Can you work these out from the model? Positions are in its coordinate system, mm. Give positions to 0.01 mm unless a question says otherwise; leave off trailing zeros. Order: outer loops, then holes, each group sorted by start corner. A loop starts at its lowest first (then second) coordinate and runs counter-clockwise, first axis right, second up. Notation, with made-up numbers: (10.5, -14.5) - (40.5, -14.5) arc R11 cw to (40.5, 0.5) - close; hole circle Ø2 at (23.25, 72). An arc over 180 degrees is marked (long way). One line per question, with ' | ' between items.
```python
from build123d import *

# Parameters (mm, degrees)
CYLINDER_R          = 1.5
CYLINDER_DEPTH      = 10
CYLINDER_ROLL_ANGLE = 90
CUT_PLACEMENT_ANGLE = 180


with BuildPart() as cylinder:
    # Cylinder → Cylinder (new body)
    with BuildSketch(Plane.XY):
        Circle(CYLINDER_R)
    extrude(amount=CYLINDER_DEPTH)


with BuildPart() as cylinder_1:
    # Cylinder roll: moved
    add(cylinder.part.rotate(Axis((0, 0, 0), (1, 0, 0)), CYLINDER_ROLL_ANGLE))


with BuildPart() as cylinder_2:
    # Cylinder placement: moved
    add(cylinder_1.part.moved(Location((0, 5, 0))))


with BuildPart() as innerbearing:
    # Sketch004 → Revolution (revolve)
    with BuildSketch(Plane.YZ):
        Polygon((0, 4.213446), (2.5, 6.311195), (2.5, 0), (0, 0), align=None)
    revolve(axis=Axis((0, 0, 0), (0, 1, 0)))

    # Cut: cut Cylinder
    add(cylinder_2.part, mode=Mode.SUBTRACT)


with BuildPart() as innerbearing_1:
    # Cut placement: moved
    add(innerbearing.part.rotate(Axis((0, 0, 0), (0, 0, 1)), CUT_PLACEMENT_ANGLE))


solid = innerbearing_1.part
```
(1) Will these pins go through, and if not, where does the flat tip stop? pin 1 (4 mm diameter, centred on x = -0.5, z = -0.5, fed in from +Y); pin 2 (1.5 mm diameter, centred on x = -1, y = -2, fed in from +Z).
Answer below:
pin 1: y = 0 | pin 2: z = 6.3
(2) If I drill on line 1 (X direction, y = -0.2, z = 1.25); line 2 (Z direction, x = 0, y = -1); line 3 (Z direction, x = 0, y = -0.75), over which ranges is the centre line in solid material (lowest first)?
Answer below:
line 1: -4.2 to -0.83, 0.83 to 4.2 | line 2: -5.05 to -1.5, 1.5 to 5.05 | line 3: -4.84 to -1.5, 1.5 to 4.84
(3) Imagine slicing it at C-C (y = -1.4). List the corners of the cut face in (x, z) for me.
Answer below:
outline: circle Ø10.78 at (0, 0); hole circle Ø3 at (0, 0)
(4) Imagine slicing it at B-B (x = 0). List the corners of the cut face in (y, z) for me, and give its area (3 significant figures).
Answer below:
outline: (-2.5, -6.31) - (0, -4.21) - (0, -1.5) - (-2.5, -1.5) - close; (-2.5, 1.5) - (0, 1.5) - (0, 4.21) - (-2.5, 6.31) - close | area: 18.8 mm^2
(5) Imagine slicing it at A-A (z = 0). List the corners of the cut face in (x, y) for me.
Answer below:
outline: (-6.31, -2.5) - (-1.5, -2.5) - (-1.5, 0) - (-4.21, 0) - close; (1.5, -2.5) - (6.31, -2.5) - (4.21, 0) - (1.5, 0) - close
(6) Imagine slicing it at D-D (y = -0.75). List the corners of the cut face in (x, z) for me, and give its area (3 significant figures).
Answer below:
outline: circle Ø9.69 at (0, 0); hole circle Ø3 at (0, 0) | area: 66.6 mm^2
(7) If we mould it in two halves opening along X, with no side actions, what happens to faces 1 (the face through (4.241, -0.156, -0.942)), 2 (the face through (0.325, -1.268, -1.464)), 3 (the face through (0, 0, -2))? For each: released by +X, released by -X, zero draft, split by the parting line, or undercut.
Answer below:
face 1: split by the parting line | face 2: undercut | face 3: zero draft
